Here's how the part is built. I have some questions about the finished solid (model axes, mm). A direction names the side the tool comes from. Coordinates: 2 decimals unless noted, no trailing zeros.
(1) Imagine slicing it at A-A, the plane z = 2.5. State how many separate pieces and enclosed holes the cut face has, plus the area to 3 significant figures.
(2) Which directions (+Z, -Z, +X, -X, +Y, -Y) give clear straight access to the entire face, cutting with the end or side of a thin tool? Please do faces 1 (the conical face through (17.75, -4.93, -0.07)), 2 (the cylindrical face through (21.156, -5.556, -0.061)), 3 (the flat face through (16.7, -0.1, -3.899)), 4 (the cylindrical face through (16.48, 4.57, 0.07)), 5 (the cylindrical face through (6.233, 0.587, -1.865)).
(3) Please list where these lines run through material, in increasing order: probe 1 along X at (y, z) = (0, 4.5); probe 2 along Z at (x, y) = (11.75, -6.75); probe 3 along Z at (x, y) = (7.25, 0).
(4) For pin 1 Ø6 at (x, y) = (9.5, 4.5) entering from +Z; pin 2 Ø3 at (x, y) = (3, 3.5) entering from -Z; pin 3 Ø6 at (x, y) = (13, 0.5) entering from +Z; pin 4 Ø2 at (x, z) = (21.5, 5.5) entering from -Y, each with a flat end and sliding along its axis, tell me the tip position at first contact or that it passes through.
(5) Thinking about a two-plate mould opening in X: for faces 6 (the flat face through (8, 2, 6.794)), 7 (the cylindrical face through (21.156, 5.556, 0.061)), 8 (the flat face through (24.613, 0, 0)), which applies, released by +X, released by -X, zero draft, split by the parting line, or undercut?
```python
from build123d import *

# Parameters (mm, degrees)
SKETCH3_W               = 31.242
SKETCH3_H               = 62.484
SKETCH3_W_2             = 7.7978
SKETCH3_H_2             = 31.242
CUT_EXTRUDE1_DEPTH      = 11.0998
HOLE1_D                 = 3.9116
HOLE1_DEPTH             = 12.2936
HOLE1_TIP               = 1.129181656
SKETCH8_R               = 2.77495
CUT_EXTRUDE2_DEPTH      = 5.84835
CUT_EXTRUDE2_DEPTH_BACK = 5.84835


with BuildPart() as part:
    # Sketch1 → Revolve1 (revolve)
    with BuildSketch(Plane.XY):
        Polygon((0, 0), (0, 6.50875), (0.762, 7.27075), (2.7178, 7.27075), (3.3528, 6.63575), (3.9878, 6.63575), (3.9878, 7.8105), (12.7508, 7.8105), (13.5128, 7.0485), (13.5128, 0), align=None)
    revolve(axis=Axis((13.5128, 0, 0), (-1, 0, 0)))

    # Sketch2 → Revolve2 (revolve)
    with BuildSketch(Plane.XY):
        with BuildLine():
            Line((13.5128, 0), (13.5128, 5.53085))
            Line((13.5128, 5.53085), (15.0876, 5.53085))
            Line((15.0876, 5.53085), (15.0876, 5.3721))
            ThreePointArc((15.0876, 5.3721), (15.321943864, 4.806343864), (15.8877, 4.572))
            Line((15.8877, 4.572), (17.0561, 4.572))
            ThreePointArc((17.0561, 4.572), (17.3228, 4.617758486), (17.558994343, 4.7498))
            Line((17.558994343, 4.7498), (17.621856136, 4.8006))
            Line((17.621856136, 4.8006), (18.377506136, 5.55625))
            Line((18.377506136, 5.55625), (23.85695, 5.55625))
            Line((23.85695, 5.55625), (24.6126, 4.8006))
            Line((24.6126, 4.8006), (24.6126, 0))
            Line((24.6126, 0), (13.5128, 0))
        make_face()
    revolve(axis=Axis((24.6126, 0, 0), (-1, 0, 0)))

    # Sketch3 → Cut-Extrude1 (cut)
    with BuildSketch(Plane(origin=(24.6126, 0, 0), x_dir=(0, 0, -1), z_dir=(1, 0, 0))):
        Rectangle(SKETCH3_W, SKETCH3_H)
        Rectangle(SKETCH3_W_2, SKETCH3_H_2, mode=Mode.SUBTRACT)
    extrude(amount=-CUT_EXTRUDE1_DEPTH, mode=Mode.SUBTRACT)

    # Hole1
    with Locations(Plane.ZY):
        with Locations((0, 0)):
            Hole(HOLE1_D / 2, depth=HOLE1_DEPTH)
            with Locations((0, 0, -(HOLE1_DEPTH + HOLE1_TIP / 2))):  # 120° drill point
                Cone(0, HOLE1_D / 2, HOLE1_TIP, mode=Mode.SUBTRACT)

    # Sketch6 → Cut-Revolve1 (revolve, cut)
    with BuildSketch(Plane(origin=(0, 0, 0), x_dir=(1, 0, 0), z_dir=(0, 1, 0))):
        Polygon((10.3124, 0), (12.29614, 0), (12.29614, -6.36524), (12.7254, -6.7945), (14.2748, -6.7945), (14.2748, -7.8105), (10.3124, -7.8105), align=None)
    revolve(axis=Axis((10.3124, 0, 7.8105), (0, 0, -1)), mode=Mode.SUBTRACT)

    # Sketch7 → Revolve3 (revolve)
    with BuildSketch(Plane.XY):
        with BuildLine():
            Line((3.160243808, 7.726331804), (3.870760245, 7.015815367))
            ThreePointArc((3.870760245, 7.015815367), (3.907957684, 6.926012806), (3.870760245, 6.836210245))
            Line((3.870760245, 6.836210245), (3.6703, 6.63575))
            Line((3.6703, 6.63575), (3.3528, 6.63575))
            Line((3.3528, 6.63575), (3.3528, 6.38175))
            Line((3.3528, 6.38175), (3.9878, 6.38175))
            Line((3.9878, 6.38175), (3.9878, 7.186143808))
            Line((3.9878, 7.186143808), (3.363443808, 7.8105))
            Line((3.363443808, 7.8105), (3.160243808, 7.8105))
            Line((3.160243808, 7.8105), (3.160243808, 7.726331804))
        make_face()
    revolve(axis=Axis((3.9878, 0, 0), (-1, 0, 0)))

    # Sketch8 → Cut-Extrude2 (cut, two sides)
    with BuildSketch(Plane.XY) as cut_extrude2_sk:
        with Locations((19.8374, 0)):
            Circle(SKETCH8_R)
    extrude(amount=CUT_EXTRUDE2_DEPTH, mode=Mode.SUBTRACT)
    extrude(cut_extrude2_sk.sketch, amount=-CUT_EXTRUDE2_DEPTH_BACK, mode=Mode.SUBTRACT)


solid = part.part
```
Recorded:
1. separate pieces: 1
1. enclosed holes: 2
1. area: 260 mm2
2. face 1: -Y
2. face 2: +X, -Y
2. face 3: -Z, +X, +Y, -Y
2. face 4: +Y
2. face 5: -X
3. probe 1: x = 0 to 8.33, 12.3 to 13.51
3. probe 2: z = -3.93 to 3.93
3. probe 3: z = -7.81 to -1.96, 1.96 to 6.79
4. pin 1: stops at z = 7.39
4. pin 2: stops at z = -7.55
4. pin 3: stops at z = 7.16
4. pin 4: passes through
5. face 6: undercut
5. face 7: zero draft
5. face 8: released by +X
